Geometry check sheet. Reference: drawing and pictorial views, mm from the part's lowest x, y, z. Round coordinates to 2 decimals unless told otherwise and drop trailing zeros. Write each loop counter-clockwise with the first axis right and the second up, starting at its lowest first coordinate (ties: lowest second). Pieces come first, ordered by that corner, then holes. Notation, with made-up numbers: (52, 14) - (64, 14) arc R32 cw to (64, 48) - close; hole circle Ø4 at (-28.75, 55). An arc over 180 degrees is marked (long way). Return JSON: item names as keys, results as strings.
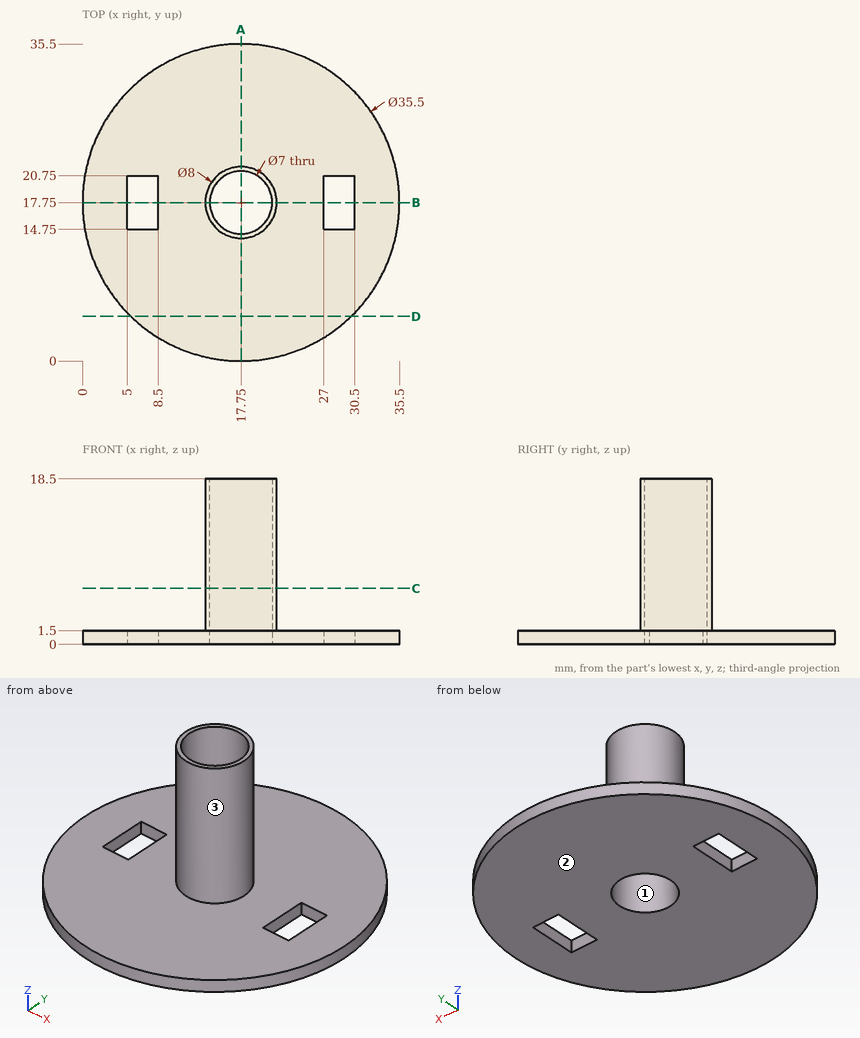
(1) Section check A-A, the plane x = 17.75. Enter the section's corners in (y, z), plus the area to 4 significant figures.
Response values:
{"outline": "(0, 0) - (14.25, 0) - (14.25, 18.5) - (13.75, 18.5) - (13.75, 1.5) - (0, 1.5) - close; (21.25, 0) - (35.5, 0) - (35.5, 1.5) - (21.75, 1.5) - (21.75, 18.5) - (21.25, 18.5) - close", "area": "59.75 mm^2"}
(2) Gauge pin test, flat ends, axial feed: pin 1 (9 mm diameter, centred on x = 17.75, y = 17.75, fed in from +Z); pin 2 (1.2 mm diameter, centred on x = 6, z = 0.5, fed in from -Y); pin 3 (0.8 mm diameter, centred on x = 29, z = 1, fed in from +Y); pin 4 (0.8 mm diameter, centred on x = 7.5, z = 0.5, fed in from +Y). Record the tip position at first contact, or that the pin passes through.
Response values:
{"pin 1": "stops at z = 18.5", "pin 2": "stops at y = 3.94", "pin 3": "stops at y = 31.8", "pin 4": "stops at y = 32.52"}
(3) Section check D-D, the plane y = 5. Enter the section's corners in (x, z).
Response values:
{"outline": "(5.4, 0) - (30.1, 0) - (30.1, 1.5) - (5.4, 1.5) - close"}
(4) Material ranges on line 1 along Y through (x, z) = (17.75, 12); line 2 along Z through (x, y) = (14, 22.5); line 3 along Y through (x, z) = (16, 6), recorded low to high. Write a range as [from, to].
Response values:
{"line 1": "y = [13.75, 14.25], [21.25, 21.75]", "line 2": "z = [0, 1.5]", "line 3": "y = [14.15, 14.72], [20.78, 21.35]"}
(5) Release check for a two-part mould opening along Y. For the marked faces 1, 2 and 3 record: pulls with the +Y half, pulls with the -Y half, needs draft (parallel to the pull), parting line crosses it, or undercut.
Response values:
{"face 1": "undercut", "face 2": "needs draft", "face 3": "parting line crosses it"}
(6) Section check B-B, the plane y = 17.75. Enter the section's corners in (x, z), plus the area to 4 significant figures.
Response values:
{"outline": "(0, 0) - (5, 0) - (5, 1.5) - (0, 1.5) - close; (8.5, 0) - (14.25, 0) - (14.25, 18.5) - (13.75, 18.5) - (13.75, 1.5) - (8.5, 1.5) - close; (21.25, 0) - (27, 0) - (27, 1.5) - (21.75, 1.5) - (21.75, 18.5) - (21.25, 18.5) - close; (30.5, 0) - (35.5, 0) - (35.5, 1.5) - (30.5, 1.5) - close", "area": "49.25 mm^2"}
(7) Section check C-C, the plane z = 6.25. Enter the section's corners in (x, y), plus the area to 3 significant figures.
Response values:
{"outline": "circle Ø8 at (17.75, 17.75); hole circle Ø7 at (17.75, 17.75)", "area": "11.8 mm^2"}
